```python
from build123d import *

# Parameters (mm, degrees)
F1_DEPTH = 561.5
F2_R     = 25
F3_DEPTH = 82.001


with BuildPart() as f1:
    # F0 (on Right) → F1 (new body, symmetric)
    with BuildSketch(Plane.YZ):
        Polygon((0, 62.5), (0, 0), (178.5, 0), (208.5, 30), (176, 62.5), (110, 62.5), (110, 82), (40, 82), (40, 62.5), align=None)
    extrude(amount=F1_DEPTH, both=True)

    # F2 (on face) → F3 (cut, through all)
    with BuildSketch(Plane.XY.offset(82)):
        with Locations((456.5, 75)):
            Circle(F2_R)
        with Locations((276.5, 75)):
            Circle(F2_R)
        with Locations((96.5, 75)):
            Circle(F2_R)
        with Locations((-83.5, 75)):
            Circle(F2_R)
        with Locations((-293.5, 75)):
            Circle(F2_R)
        with Locations((-473.5, 75)):
            Circle(F2_R)
    extrude(amount=-F3_DEPTH, mode=Mode.SUBTRACT)


solid = f1.part
```
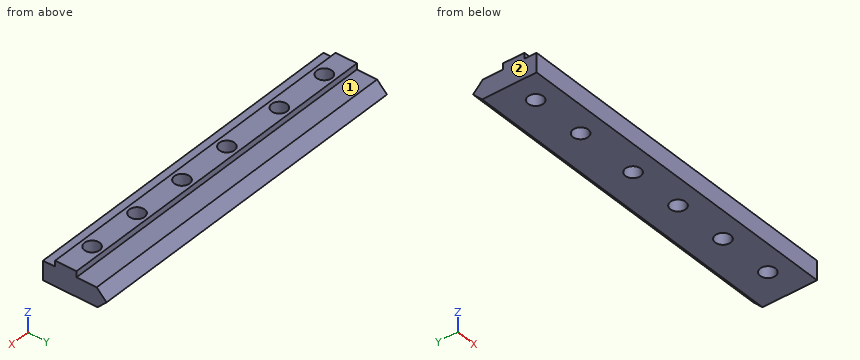
Could you check a few things on this model? Use its own coordinates, in mm. Face numbers are marked on the shaded views. A direction names the side the tool comes from. Give positions to 0.01 mm unless a question says otherwise; leave off trailing zeros. Loops run counter-clockwise (first coordinate to the right, second up) from the corner with the lowest first, then second, coordinate; pieces in that order, holes last. Notation, with made-up numbers: (67, 76) - (88, 76) arc R18 cw to (88, 93) - close; hole circle Ø10 at (38.5, -22.5). An arc over 180 degrees is marked (long way). Answer in a Markdown table with one row per item. Add a question column.
Q1. If we section it at D-D (y = 135.5): List the corners of the cut face in (x, z) for me, plus the area to 3 significant figures.
Q2. If we section it at C-C (x = 224): List the corners of the cut face in (y, z) for me, plus the area to 3 significant figures.
Q3. If we section it at A-A (y = 75): List the corners of the cut face in (x, z) for me.
Q4. If we section it at B-B (x = 456.5): List the corners of the cut face in (y, z) for me.
Q5. Please list where these lines run through material, in increasing order: L1, parallel to Y at x = -473, z = 30 (3 decimals); L2, parallel to Z at x = 27.5, y = 120.5; L3, parallel to Y at x = -472, z = 72. Write a range as from..to.
Q6. For pin 1 (20 mm diameter, centred on x = -183.5, y = 135, fed in from +Z); pin 2 (4 mm diameter, centred on x = 417.5, z = 50, fed in from -Y); pin 3 (10 mm diameter, centred on x = -145, z = 71, fed in from -Y); pin 4 (4 mm diameter, centred on x = -20.5, z = 30.5, fed in from +Y), each with a flat end and sliding along its axis, tell me the tip position at first contact or that it passes through.
Q7. Which directions (+Z, -Z, +X, -X, +Y, -Y) give clear straight access to the entire face, cutting with the end or side of a thin tool? Please do the marked faces 1 and 2.
The answers:
| question | item | result |
|---|---|---|
| 1 | outline | (-561.5, 0) - (561.5, 0) - (561.5, 62.5) - (-561.5, 62.5) - close |
| 1 | area | 70,200 mm^2 |
| 2 | outline | (0, 0) - (178.5, 0) - (208.5, 30) - (176, 62.5) - (110, 62.5) - (110, 82) - (40, 82) - (40, 62.5) - (0, 62.5) - close |
| 2 | area | 13,400 mm^2 |
| 3 | outline | (-561.5, 0) - (-498.5, 0) - (-498.5, 82) - (-561.5, 82) - close; (-448.5, 0) - (-318.5, 0) - (-318.5, 82) - (-448.5, 82) - close; (-268.5, 0) - (-108.5, 0) - (-108.5, 82) - (-268.5, 82) - close; (-58.5, 0) - (71.5, 0) - (71.5, 82) - (-58.5, 82) - close; (121.5, 0) - (251.5, 0) - (251.5, 82) - (121.5, 82) - close; (301.5, 0) - (431.5, 0) - (431.5, 82) - (301.5, 82) - close; (481.5, 0) - (561.5, 0) - (561.5, 82) - (481.5, 82) - close |
| 4 | outline | (0, 0) - (50, 0) - (50, 82) - (40, 82) - (40, 62.5) - (0, 62.5) - close; (100, 0) - (178.5, 0) - (208.5, 30) - (176, 62.5) - (110, 62.5) - (110, 82) - (100, 82) - close |
| 5 | L1 | y = 0..50.005, 99.995..208.5 |
| 5 | L2 | z = 0..62.5 |
| 5 | L3 | y = 40..50.05, 99.95..110 |
| 6 | pin 1 | stops at z = 62.5 |
| 6 | pin 2 | stops at y = 0 |
| 6 | pin 3 | stops at y = 40 |
| 6 | pin 4 | stops at y = 208.5 |
| 7 | face 1 | +Z, +X, -X, +Y |
| 7 | face 2 | +Z, -Z, -X, +Y, -Y |
